```python
from build123d import *

# Parameters (mm, degrees)
SKETCH_1_R      = 7
EXTRUDE_1_DEPTH = 12


with BuildPart() as part:
    # 草图1 → 凸台-拉伸1 (new body)
    with BuildSketch(Plane.XY):
        Polygon((5.484827557, 9.5), (-5.484827557, 9.5), (-10.969655115, 0), (-5.484827557, -9.5), (5.484827557, -9.5), (10.969655115, 0), align=None)
        Circle(SKETCH_1_R, mode=Mode.SUBTRACT)
    extrude(amount=EXTRUDE_1_DEPTH)

    # 草图2 → 旋转1 (revolve)
    with BuildSketch(Plane(origin=(0, 0, 0), x_dir=(1, 0, 0), z_dir=(0, 1, 0)), mode=Mode.PRIVATE) as revolve_1_sk:
        Polygon((-7.15, 0), (-7.15, 2), (-6.55, 7.8), (-7.15, 7.8), (-7.15, 9.3), (-6.55, 14.3), (-7.15, 14.3), (-7.15, 15.8), (-6.55, 20.8), (-7.15, 20.8), (-7.15, 24), (-6, 24), (-6, 0), align=None)
    revolve(revolve_1_sk.sketch.rotate(Axis((0, 0, 0), (0, 0, -1)), 180), axis=Axis((0, 0, 0), (0, 0, -1)))


solid = part.part
```
Verification items for the finished model (mm, model axes). A direction names the side the tool comes from. Give positions to 0.01 mm unless a question says otherwise; leave off trailing zeros. Order: outer loops, then holes, each group sorted by start corner. A loop starts at its lowest first (then second) coordinate and runs counter-clockwise, first axis right, second up. Notation, with made-up numbers: M 2.5,-9 L 21.5,-9 A21 cw 21.5,1 Z; hole C 27,50.25 d1. An arc over 180 degrees is marked long. Return JSON: item names as keys, results as strings. Group by question number.
1) Section check C-C on x = -9. Record the cut outline in (y, z), and give its area (3 significant figures).
2) Mould release check, pull along X, two halves, no side actions. Record for faces 1 (the face through (-6, -2, 0)), 2 (the face through (6.466, -2.681, 5.916)), 3 (the face through (8.266, 4.684, 5.916)), 4 (the face through (6.466, -2.036, -5.585)): pulls with the +X half, pulls with the -X half, needs draft (parallel to the pull), parting line crosses it, or undercut.
3) Go/stop test with flat-tipped pins: pin 1 Ø4 at (x, z) = (5.5, -8) entering from +Y; pin 2 Ø1 at (x, z) = (6.5, -16.5) entering from -Y; pin 3 Ø5 at (x, z) = (-7.5, -18.5) entering from -Y. Record where each tip stops, or that it passes through.
4) Scan lines: line 1 (Y direction, x = 0, z = 6.75); line 2 (Y direction, x = 0, z = -8.5); line 3 (X direction, y = 2.25, z = -19). Record each from-to range of solid material in increasing order.
5) Section check A-A on z = 0.5. Record the cut outline in (x, y), and give its area (3 significant figures).
6) Access from +Z, -Z, +X, -X, +Y, -Y to the whole of each face (thin tool, end or side, straight path). Record for faces 5 (the face through (-1.47, 6.618, -18.891)), 6 (the face through (7.2, 0.1, 12)), 7 (the face through (-0.93, -7.09, -8.56)).
Answer block:
{
 "1": {"outline": "M -3.41,0 L 3.41,0 L 3.41,12 L -3.41,12 Z", "area": "81.9 mm^2"},
 "2": {"face 1": "undercut", "face 2": "undercut", "face 3": "pulls with the +X half", "face 4": "parting line crosses it"},
 "3": {"pin 1": "stops at y = 6.23", "pin 2": "stops at y = -3.74", "pin 3": "stops at y = -4.68"},
 "4": {"line 1": "y = -9.5 to -7, 7 to 9.5", "line 2": "y = -7.15 to -6, 6 to 7.15", "line 3": "x = -6.38 to -5.56, 5.56 to 6.38"},
 "5": {"outline": "M -10.97,0 L -5.48,-9.5 L 5.48,-9.5 L 10.97,0 L 5.48,9.5 L -5.48,9.5 Z; hole C 0,0 d14", "area": "159 mm^2"},
 "6": {"face 5": "none", "face 6": "+Z, +X, -X, +Y, -Y", "face 7": "-Z"}
}
